```python
from build123d import *

# Parameters (mm, degrees)
F0_R     = 11
F1_DEPTH = 6.5
F2_R     = 3
F3_R     = 3


with BuildPart() as f1:
    # F0 (on Front) → F1 (new body)
    with BuildSketch(Plane.XZ):
        with BuildLine():
            ThreePointArc((8.740666, -15.348029), (15.269948, -8.87637), (17.662425, 0))
            ThreePointArc((17.662425, 0), (17.658261, 0.383509), (17.64577, 0.766837))
            ThreePointArc((17.64577, 0.766837), (15.127751, 9.1166), (8.92145, 15.243654))
            ThreePointArc((8.92145, 15.243654), (-0.331332, 17.659317), (-9.486986, 14.898267))
            ThreePointArc((-9.486986, 14.898267), (-15.459083, 8.542717), (-17.662116, 0.104376))
            ThreePointArc((-17.662116, 0.104376), (-15.127751, -9.1166), (-8.158784, -15.665104))
            ThreePointArc((-8.158784, -15.665104), (0.331332, -17.659317), (8.740666, -15.348029))
        make_face()
        Circle(F0_R, mode=Mode.SUBTRACT)
        with BuildLine():
            ThreePointArc((17.64577, 0.766837), (17.658261, 0.383509), (17.662425, 0))
            ThreePointArc((17.662425, 0), (15.269948, -8.87637), (8.740666, -15.348029))
            Line((8.740666, -15.348029), (12.508677, -17.523491))
            Line((12.508677, -17.523491), (9.359866, -22.977391))
            Line((9.359866, -22.977391), (55.553557, -32.073861))
            Line((55.553557, -32.073861), (24.805502, 4.744098))
            Line((24.805502, 4.744098), (21.293365, -1.339102))
            Line((21.293365, -1.339102), (17.64577, 0.766837))
        make_face()
        with BuildLine():
            ThreePointArc((-9.486986, 14.898267), (-0.331332, 17.659317), (8.92145, 15.243654))
            Line((8.92145, 15.243654), (8.92145, 19.594578))
            Line((8.92145, 19.594578), (15.219072, 19.594578))
            Line((15.219072, 19.594578), (0, 64.147722))
            Line((0, 64.147722), (-16.51126, 19.110146))
            Line((-16.51126, 19.110146), (-9.486986, 19.110146))
            Line((-9.486986, 19.110146), (-9.486986, 14.898267))
        make_face()
        with BuildLine():
            Line((-11.806379, -17.771044), (-8.158784, -15.665104))
            ThreePointArc((-8.158784, -15.665104), (-15.127751, -9.1166), (-17.662116, 0.104376))
            Line((-17.662116, 0.104376), (-21.430127, -2.071086))
            Line((-21.430127, -2.071086), (-24.578938, 3.382814))
            Line((-24.578938, 3.382814), (-55.553557, -32.073861))
            Line((-55.553557, -32.073861), (-8.294242, -23.854243))
            Line((-8.294242, -23.854243), (-11.806379, -17.771044))
        make_face()
    extrude(amount=F1_DEPTH)

    # F2
    f2_edges = [f1.edges().sort_by_distance(p)[0] for p in [
        (-8.25563, -6.5, 41.628934),
        (7.609536, -6.5, 41.87115),
        (40.179529, -6.5, -13.664882),
        (32.456712, -6.5, -27.525626),
        (-31.923899, -6.5, -27.964052),
        (-40.066247, -6.5, -14.345524),
    ]]
    fillet(f2_edges, radius=F2_R)

    # F3
    f3_edges = [f1.edges().sort_by_distance(p)[0] for p in [
        (40.179529, 0, -13.664882),
        (-31.923899, 0, -27.964052),
        (32.456712, 0, -27.525626),
        (-40.066247, 0, -14.345524),
        (-8.25563, 0, 41.628934),
        (7.609536, 0, 41.87115),
    ]]
    fillet(f3_edges, radius=F3_R)


solid = f1.part
```
Work out the finished part from the listing and answer in its coordinate system (mm). A direction names the side the tool comes from. Coordinates: 2 decimals unless noted, no trailing zeros. Write each loop counter-clockwise with the first axis right and the second up, starting at its lowest first coordinate (ties: lowest second). Pieces come first, ordered by that corner, then holes. Notation, with made-up numbers: (56, -39) - (113, -39) arc R22 ccw to (113, -8) - close; hole circle Ø2 at (29, -17). An arc over 180 degrees is marked (long way). Answer as a JSON object with one key per item and string values.
Q1. For a pull along X with two mould halves and no side action, classify faces 4 (the flat face through (-4, 0, -11)), 5 (the cylindrical face through (-39.64, -5.6, -15.16)), 6 (the flat face through (19.495, -3.204, -0.301)), 7 (the cylindrical face through (-2.38, -3.2, -10.74)) as pulls with the +X half, pulls with the -X half, needs draft (parallel to the pull), parting line crosses it, or undercut.
Results list:
{"face 4": "needs draft", "face 5": "pulls with the -X half", "face 6": "undercut", "face 7": "undercut"}
Q2. Consider L1, parallel to X at y = -5.5, z = -5; L2, parallel to X at y = -2, z = -9.5; L3, parallel to X at y = -3.5, z = 11.5. Determine where each line is inside the solid, lowest interval first. Write a range as from..to.
Results list:
{"L1": "x = -30.89..-9.8, 9.8..31.95", "L2": "x = -35.61..-5.55, 5.55..36.48", "L3": "x = -13.41..13.41"}
Q3. Given pin 1 Ø1 at (x, y) = (-26, -5) entering from -Z; pin 2 Ø1 at (y, z) = (-5.5, 25) entering from -X; pin 3 Ø1.5 at (x, y) = (16.5, -4.5) entering from -Z, each flat-ended and moving along its own axis, determine where each tip first touches the part or whether it passes through.
Results list:
{"pin 1": "stops at z = -26.78", "pin 2": "stops at x = -13.97", "pin 3": "stops at z = -24.45"}
Q4. Find section A-A (y = -1.5). Write down the section's boundary in (x, z) (1 decimal).
Results list:
{"outline": "(-54.5, -31.5) - (-8.5, -23.5) - (-11.8, -17.8) - (-8.2, -15.7) arc R17.7 ccw to (8.7, -15.3) - (12.5, -17.5) - (9.6, -22.6) - (54.5, -31.5) - (24.6, 4.4) - (21.3, -1.3) - (17.6, 0.8) arc R17.7 ccw to (8.9, 15.2) - (8.9, 19.6) - (14.8, 19.6) - (0, 62.9) - (-16.1, 19.1) - (-9.5, 19.1) - (-9.5, 14.9) arc R17.7 ccw to (-17.7, 0.1) - (-21.4, -2.1) - (-24.4, 3) - close; hole circle Ø22 at (0, 0)"}
Q5. Which of the six approach directions +Z, -Z, +X, -X, +Y, -Y give full straight-line access (tool end or side, diameter ignored) to faces 1 (the cylindrical face through (32.95, -5.6, -26.75)), 2 (the flat face through (-22.982, -3.204, 0.618)), 3 (the cylindrical face through (32.95, -0.9, -26.75))?
Results list:
{"face 1": "-Z, -Y", "face 2": "+Z, +Y, -Y", "face 3": "-Z, +Y"}
